```python
from build123d import *

# Parameters (mm, degrees)
SKETCH1_R           = 7.5
SKETCH1_R_2         = 3.5
BOSS_EXTRUDE1_DEPTH = 11
CHAMFER1_SIZE       = 1
CHAMFER2_SIZE       = 1.5


with BuildPart() as part:
    # Sketch1 → Boss-Extrude1 (new body)
    with BuildSketch(Plane(origin=(0, 0, 0), x_dir=(1, 0, 0), z_dir=(0, 1, 0))):
        with Locations(Location((0, 0, 0), (0, 0, 270))):
            Circle(SKETCH1_R)
        with Locations(Location((0, 0, 0), (0, 0, 270))):
            Circle(SKETCH1_R_2, mode=Mode.SUBTRACT)
    extrude(amount=BOSS_EXTRUDE1_DEPTH)

    # Chamfer1
    chamfer1_edges = [part.edges().sort_by_distance(p)[0] for p in [
        (0, 0, -3.5),
    ]]
    chamfer(chamfer1_edges, length=CHAMFER1_SIZE)

    # Chamfer2
    chamfer2_edges = [part.edges().sort_by_distance(p)[0] for p in [
        (0, 0, -7.5),
        (0, 11, -7.5),
    ]]
    chamfer(chamfer2_edges, length=CHAMFER2_SIZE)


solid = part.part
```
Part model, mm, in its own coordinate system. Round coordinates to 2 decimals unless told otherwise and drop trailing zeros. Loops run counter-clockwise (first coordinate to the right, second up) from the corner with the lowest first, then second, coordinate; pieces in that order, holes last. Notation, with made-up numbers: (-23.75, 32) -> (35.25, 32) arc R12 ccw to (35.25, 55) -> close; hole circle Ø1 at (0.25, 43.5). An arc over 180 degrees is marked (long way). Use one line per item in the form item = value. Start each with the question number.
Item 1: Band-saw the part on B-B (x = 0). List the corners of the cut face in (y, z), plus the area to 3 significant figures.
Item 2: Band-saw the part on C-C (y = 3.5). List the corners of the cut face in (x, z).
Item 3: Drill centre lines: line 1 along X through (y, z) = (3.5, 0); line 2 along Z through (x, y) = (-1.75, 9); line 3 along Z through (x, y) = (-1.5, 0.75). Where is each one in solid material? Low to high.
Item 4: Two-plate mould, pull along X, no slides. Class faces 1 (the flat face through (4.5, 0, -1.4)), 2 (the cylindrical face through (0.33, 5.444, -7.493)), 3 (the cylindrical face through (-3.417, 5.93, -0.759)): released by +X, released by -X, zero draft, split by the parting line, or undercut.
Item 5: Band-saw the part on A-A (z = 0). List the corners of the cut face in (x, y), plus the area to 3 significant figures.
Item 6: Drop flat-ended pins along their axis: pin 1 Ø6 at (x, z) = (-4.5, -4.5) entering from +Y; pin 2 Ø1.5 at (y, z) = (5, -1) entering from -X; pin 3 Ø1.5 at (y, z) = (9, 3.5) entering from +X; pin 4 Ø6 at (y, z) = (8.5, -4) entering from -X. Give the stop position or say it passes through.
Data:
q1.outline = (0, -6) -> (1.5, -7.5) -> (9.5, -7.5) -> (11, -6) -> (11, -3.5) -> (1, -3.5) -> (0, -4.5) -> close; (0, 4.5) -> (1, 3.5) -> (11, 3.5) -> (11, 6) -> (9.5, 7.5) -> (1.5, 7.5) -> (0, 6) -> close
q1.area = 82.5 mm^2
q2.outline = circle Ø15 at (0, 0); hole circle Ø7 at (0, 0)
q3.line_1 = -7.5 to -3.5, 3.5 to 7.5
q3.line_2 = -7.29 to -3.03, 3.03 to 7.29
q3.line_3 = -6.58 to -3.44, 3.44 to 6.58
q4.face_1 = zero draft
q4.face_2 = split by the parting line
q4.face_3 = undercut
q5.outline = (-7.5, 1.5) -> (-6, 0) -> (-4.5, 0) -> (-3.5, 1) -> (-3.5, 11) -> (-6, 11) -> (-7.5, 9.5) -> close; (3.5, 1) -> (4.5, 0) -> (6, 0) -> (7.5, 1.5) -> (7.5, 9.5) -> (6, 11) -> (3.5, 11) -> close
q5.area = 82.5 mm^2
q6.pin_1 = 11
q6.pin_2 = -7.5
q6.pin_3 = 6.98
q6.pin_4 = -7.43
